from build123d import *

# Parameters (mm, degrees)
BOSS_EXTRUDE2_DEPTH     = 10
CUT_EXTRUDE2_REACH      = 236.376
SKETCH2_R               = 4.5
SKETCH3_R               = 9.5
CUT_EXTRUDE3_DEPTH      = 6
SKETCH6_W               = 24.299182762
SKETCH6_H               = 10
SKETCH6_W_2             = 24.299182761
BOSS_EXTRUDE7_DEPTH     = 15
CUT_EXTRUDE5_DEPTH      = 15
CUT_EXTRUDE5_DEPTH_BACK = 10
SKETCH5_R               = 2
SKETCH10_W              = 65
SKETCH10_H              = 35
CUT_EXTRUDE6_DEPTH      = 235.64297264
SKETCH11_R              = 4.5
SKETCH11_W              = 65
SKETCH11_H              = 35
BOSS_EXTRUDE8_DEPTH     = 10
SKETCH12_R              = 50
BOSS_EXTRUDE9_DEPTH     = 10
SKETCH13_R              = 3
CUT_EXTRUDE7_DEPTH      = 10
BOSS_EXTRUDE10_START    = 15
SKETCH14_R              = 12.5
SKETCH14_R_2            = 3
BOSS_EXTRUDE10_DEPTH    = 15
CUT_EXTRUDE8_START      = -6
SKETCH15_R              = 9.5
CUT_EXTRUDE8_DEPTH      = 6


with BuildPart() as part:
    # Sketch1 → Boss-Extrude2 (new body)
    with BuildSketch(Plane.XY):
        with BuildLine():
            Line((-99.83076192, 169.92150388), (-144.590341361, 91.840904188))
            ThreePointArc((-144.590341361, 91.840904188), (-144.536211539, 68.422267368), (-124.24600733, 56.7285471))
            Line((-124.24600733, 56.7285471), (-79.486427889, 56.7285471))
            Line((-79.486427889, 56.7285471), (-79.24600733, 56.7285471))
            Line((-79.24600733, 56.7285471), (-56.036427889, 56.7285471))
            Line((-56.036427889, 56.7285471), (-56.036427889, 158.259146792))
            ThreePointArc((-56.036427889, 158.259146792), (-73.452032021, 180.919432901), (-99.83076192, 169.92150388))
        make_face()
    extrude(amount=BOSS_EXTRUDE2_DEPTH)

    # Sketch2 → Cut-Extrude2 (cut, up to next)
    with BuildSketch(Plane.XY.offset(10), mode=Mode.PRIVATE) as cut_extrude2_sk1:
        with Locations((-79.486427889, 158.259146792)):
            Circle(SKETCH2_R)
    cut_extrude2_tool1 = extrude(cut_extrude2_sk1.sketch, amount=-CUT_EXTRUDE2_REACH, mode=Mode.PRIVATE) & part.part
    add(cut_extrude2_tool1.solids().sort_by_distance((-79.486428, 158.259147, 10))[0], mode=Mode.SUBTRACT)

    # Sketch3 → Cut-Extrude3 (cut)
    with BuildSketch(Plane.XY.offset(10)):
        with Locations((-79.486427889, 158.259146792)):
            Circle(SKETCH3_R)
    extrude(amount=-CUT_EXTRUDE3_DEPTH, mode=Mode.SUBTRACT)

    # Sketch6 → Boss-Extrude7 (add)
    with BuildSketch(Plane.XY.offset(10)):
        with Locations((-79.278789724, 123.259146792)):
            Rectangle(SKETCH6_W, SKETCH6_H)
        with Locations((-79.064929675, 172.759146792)):
            Rectangle(SKETCH6_W_2, SKETCH6_H)
    extrude(amount=BOSS_EXTRUDE7_DEPTH)

    # Sketch5 → Cut-Extrude5 (cut, two sides: drawn at the far end of the back side and taken through both)
    with BuildSketch(Plane.XY.offset(10).offset(-CUT_EXTRUDE5_DEPTH_BACK)):
        with Locations((-84.486427889, 172.259146792)):
            Circle(SKETCH5_R)
        with Locations((-74.486427889, 172.259146792)):
            Circle(SKETCH5_R)
        with Locations((-84.486427889, 123.259146792)):
            Circle(SKETCH5_R)
        with Locations((-74.486427889, 123.259146792)):
            Circle(SKETCH5_R)
    extrude(amount=CUT_EXTRUDE5_DEPTH + CUT_EXTRUDE5_DEPTH_BACK, mode=Mode.SUBTRACT)

    # Sketch10 → Cut-Extrude6 (cut, through all)
    with BuildSketch(Plane.XY.offset(10)):
        with Locations((-95.536427889, 84.2285471)):
            Rectangle(SKETCH10_W, SKETCH10_H)
    extrude(amount=-CUT_EXTRUDE6_DEPTH, mode=Mode.SUBTRACT)



with BuildPart() as body_2:
    # Sketch11 → Boss-Extrude8 (new body)
    with BuildSketch(Plane(origin=(0, 0, -40), x_dir=(-1, 0, 0), z_dir=(0, 0, -1))):
        with BuildLine():
            Line((56.036427889, 56.7285471), (56.036427889, 158.259146792))
            ThreePointArc((56.036427889, 158.259146792), (71.460186532, 180.292801725), (97.442137883, 173.342083462))
            Line((97.442137883, 173.342083462), (144.590341361, 91.840904188))
            ThreePointArc((144.590341361, 91.840904188), (144.582356287, 68.395530793), (124.24600733, 56.7285471))
            Line((124.24600733, 56.7285471), (56.036427889, 56.7285471))
        make_face()
        with Locations(Location((79.486427889, 158.259146792, 0), (0, 0, 180))):
            Circle(SKETCH11_R, mode=Mode.SUBTRACT)
        with Locations((95.536427889, 84.2285471)):
            Rectangle(SKETCH11_W, SKETCH11_H, mode=Mode.SUBTRACT)
    extrude(amount=BOSS_EXTRUDE8_DEPTH)


with BuildPart() as part_1:
    add(part.part)

    add(body_2.part)  # Boss-Extrude9 merges body 2
    # Sketch12 → Boss-Extrude9 (add)
    with BuildSketch(Plane.XZ.offset(-56.7285471)):
        with Locations(Location((-96.036427889, -20, 0), (0, 0, 36.869897646))):
            Circle(SKETCH12_R)
    extrude(amount=BOSS_EXTRUDE9_DEPTH)

    # Sketch13 → Cut-Extrude7 (cut)
    with BuildSketch(Plane(origin=(0, 56.7285471, 0), x_dir=(1, 0, 0), z_dir=(0, 1, 0))):
        with Locations(Location((-96.036427889, 20, 0), (0, 0, 270))):
            Circle(SKETCH13_R)
    extrude(amount=-CUT_EXTRUDE7_DEPTH, mode=Mode.SUBTRACT)

    # Sketch14 → Boss-Extrude10 (add)
    with BuildSketch(Plane(origin=(0, 56.7285471, 0), x_dir=(1, 0, 0), z_dir=(0, 1, 0)).offset(BOSS_EXTRUDE10_START)):
        with Locations(Location((-96.036427889, 20, 0), (0, 0, 90))):
            Circle(SKETCH14_R)
        with Locations(Location((-96.036427889, 20, 0), (0, 0, 270))):
            Circle(SKETCH14_R_2, mode=Mode.SUBTRACT)
    extrude(amount=-BOSS_EXTRUDE10_DEPTH)

    # Sketch15 → Cut-Extrude8 (cut)
    with BuildSketch(Plane(origin=(0, 0, -50), x_dir=(-1, 0, 0), z_dir=(0, 0, -1)).offset(CUT_EXTRUDE8_START)):
        with Locations(Location((79.486427889, 158.259146792, 0), (0, 0, 180))):
            Circle(SKETCH15_R)
    extrude(amount=CUT_EXTRUDE8_DEPTH, mode=Mode.SUBTRACT)


solid = part_1.part
Input: part model. Units: mm. Frame: model coordinates. A direction names the side the tool comes from. Give positions to 0.01 mm unless a question says otherwise; leave off trailing zeros. Write each loop counter-clockwise with the first axis right and the second up, starting at its lowest first coordinate (ties: lowest second). Pieces come first, ordered by that corner, then holes. Notation, with made-up numbers: (9.5, 53) -> (55.5, 53) arc R14 cw to (55.5, 65) -> close; hole circle Ø9 at (84, -33). An arc over 180 degrees is marked (long way). Use one line per item in the form item = value. Start each with the question number.
1) Ray query, probe 1 along Z at (x, y) = (-57.5, 69); probe 2 along Z at (x, y) = (-105, 58); probe 3 along Z at (x, y) = (-105.5, 63). Return the intervals inside material, ascending. Write a range as from..to.
2) Set-up query: faces 5 (the flat face through (-63.036, 84, -45)), 6 (the flat face through (-56.036, 107, -45)), 7 (the flat face through (-66.915, 173, 17)), 8 (the cylindrical face through (-82.64, 122.49, 12.32)), 9 (the flat face through (-120.686, 133.162, -44.93)). Return all of +Z, -Z, +X, -X, +Y, -Y with unobstructed straight access to the full face (end or side cutting, diameter ignored); none if empty.
3) Section query C-C on x = -121. Return the cut outline in (y, z), then the cut area to 3 significant figures.
4) Section query A-A on y = 62.5. Return the cut outline in (x, z).
5) Draft query along Z for faces 1 (the flat face through (-92, 120, -50)), 2 (the flat face through (-79, 173, 25)), 3 (the cylindrical face through (-93.06, 59.4, -20.39)), 4 (the flat face through (-79, 177.759, 17)). Return one class per face: pulls with the +Z half, pulls with the -Z half, needs draft (parallel to the pull), parting line crosses it, or undercut.
6) Section query B-B on z = -20. Return the cut outline in (x, y).
7) Section query D-D on y = 85.5. Return the cut outline in (x, z).
8) Pin query (flat end, axial travel): pin 1 (8 mm diameter, centred on y = 88.5, z = -46, fed in from -X); pin 2 (5 mm diameter, centred on x = -132.5, y = 109, fed in from +Z); pin 3 (11 mm diameter, centred on x = -102, z = -42.5, fed in from +Y). Return the tip coordinate at first contact, or that it passes through.
Outcome:
q1.probe_1 = -50..-40, 0..10
q1.probe_2 = -50..-40, -28.71..-11.29, 0..10
q1.probe_3 = -50..-40, -28.17..-11.83, 0..10
q2.face_5 = +Z, -Z
q2.face_6 = +Z, -Z, +X, +Y
q2.face_7 = +Z, +X, +Y
q2.face_8 = +Z
q2.face_9 = -Z, -X, +Y
q3.outline = (46.73, -63.32) -> (56.73, -63.32) -> (56.73, -50) -> (66.73, -50) -> (66.73, -40) -> (56.73, -40) -> (56.73, 0) -> (66.73, 0) -> (66.73, 10) -> (56.73, 10) -> (56.73, 23.32) -> (46.73, 23.32) -> close; (101.73, -50) -> (132.62, -50) -> (132.62, -40) -> (101.73, -40) -> close; (101.73, 0) -> (132.99, 0) -> (132.99, 10) -> (101.73, 10) -> close
q3.area = 1,690 mm^2
q4.outline = (-139.73, -50) -> (-56.04, -50) -> (-56.04, -40) -> (-139.73, -40) -> close; (-139.65, 0) -> (-56.04, 0) -> (-56.04, 10) -> (-139.65, 10) -> close; circle Ø25 at (-96.04, -20); hole circle Ø6 at (-96.04, -20)
q5.face_1 = pulls with the -Z half
q5.face_2 = pulls with the +Z half
q5.face_3 = undercut
q5.face_4 = needs draft
q6.outline = (-146.04, 46.73) -> (-99.04, 46.73) -> (-99.04, 71.73) -> (-108.54, 71.73) -> (-108.54, 56.73) -> (-146.04, 56.73) -> close; (-93.04, 46.73) -> (-46.04, 46.73) -> (-46.04, 56.73) -> (-83.54, 56.73) -> (-83.54, 71.73) -> (-93.04, 71.73) -> close
q7.outline = (-147.11, -50) -> (-128.04, -50) -> (-128.04, -40) -> (-147.11, -40) -> close; (-147.08, 0) -> (-128.04, 0) -> (-128.04, 10) -> (-147.08, 10) -> close; (-63.04, -50) -> (-56.04, -50) -> (-56.04, -40) -> (-63.04, -40) -> close; (-63.04, 0) -> (-56.04, 0) -> (-56.04, 10) -> (-63.04, 10) -> close
q8.pin_1 = -147.32
q8.pin_2 = 10
q8.pin_3 = 174.4
